Autodesk Inventor part; units mm, degrees
ref_plane "YZ Plane" through (0, 0, 0) normal (1, 0, 0) x (0, 1, 0)
ref_plane "XZ Plane" through (0, 0, 0) normal (0, 1, 0) x (-1, 0, 0)
ref_plane "XY Plane" through (0, 0, 0) normal (0, 0, 1) x (1, 0, 0)
sketch "Sketch1" plane through (0, 0, 0) normal (0, 1, 0) x (-1, 0, 0)
  line L0 (0, 0) -> (0, -71.12)
  line L1 (0, -71.12) -> (71.12, -71.12)
  line L2 (71.12, -71.12) -> (71.12, 0)
  line L3 (71.12, 0) -> (0, 0)
  arc A0 (71.12, -71.12) -> (71.12, 0) centre (-71.8439, -35.56) ccw
  arc A1 (0, 0) -> (0, -71.12) centre (142.9639, -35.56) ccw
  arc A2 (0, -71.12) -> (71.12, -71.12) centre (35.56, 71.8439) ccw
  arc A3 (71.12, 0) -> (0, 0) centre (35.56, -142.9639) ccw
  circle A4 centre (35.56, -35.56) radius 24.13
  dimension "d9" = 71.12
  dimension "d10" = 71.12
  dimension "d14" = 147.32
  dimension "d17" = 48.26
  dimension "d18" = 35.56
  dimension "d19" = 35.56
extrude "Extrusion1" add sketch "Sketch1" along normal blind 3.81
fillet "Fillet1" radius 3.175 4 edges at (0, 1.905, 0) (0, 1.905, -71.12) (-71.12, 1.905, 0) (-71.12, 1.905, -71.12)
sketch "Sketch2" plane through (0, 3.81, 0) normal (0, 1, 0) x (1, 0, 0)
  point P0 (0, 0)
sketch "Sketch3" plane through (0, 0, 0) normal (0, -1, 0) x (1, 0, 0)
  circle A0 centre (-35.56, -35.56) radius 24.13
  circle A1 centre (-35.56, -35.56) radius 31.75
  circle A2 centre (-35.56, -35.56) radius 24.13
  point P0 (0, 0)
  dimension "d23" = 63.5
extrude "Extrusion2" cut sketch "Sketch3" against normal blind 2.1079
sketch "Sketch4" plane through (0, 0, 0) normal (0, -1, 0) x (1, 0, 0)
  circle A0 centre (-35.56, -35.56) radius 24.13
  circle A1 centre (-35.56, -35.56) radius 31.75
  circle A2 centre (-60.96, -10.16) radius 1.905
  arc A3 (-1.9053, 0.4605) -> (-69.2147, 0.4605) centre (-35.56, -142.9639) ccw construction
  line L0 (-35.56, 4.3561) -> (-35.56, -75.4761) construction
  arc A4 (-69.2147, -71.5805) -> (-1.9053, -71.5805) centre (-35.56, 71.8439) ccw construction
  arc A5 (-71.5805, -1.9053) -> (-71.5805, -69.2147) centre (71.8439, -35.56) ccw construction
  line L1 (-75.4761, -35.56) -> (4.3561, -35.56) construction
  arc A6 (0.4605, -69.2147) -> (0.4605, -1.9053) centre (-142.9639, -35.56) ccw construction
  line L2 (-75.4761, -35.56) -> (-75.4761, 1.4435) construction
  circle A7 centre (-10.16, -10.16) radius 1.905
  line L3 (4.3561, -35.56) -> (4.3561, 1.4435) construction
  circle A8 centre (-60.96, -60.96) radius 1.905
  circle A9 centre (-10.16, -60.96) radius 1.905
  point P0 (0, 0)
  dimension "d26" = 3.81
  dimension "d34" = 25.4
  dimension "d35" = 25.4
  dimension "d36" = 14.5161
  dimension "d37" = 14.5162
  dimension "d38" = 50.8
  dimension "d39" = 50.8
extrude "Extrusion3" cut sketch "Sketch4" against normal blind 25.4 contours A2 | A7 | A8 | A9
sketch "Sketch6" plane through (0, 0, 0) normal (0, -1, 0) x (1, 0, 0)
  point P0 (0, 0)
sketch "Sketch8" plane through (0, 3.81, 0) normal (0, 1, 0) x (1, 0, 0)
  circle A0 centre (-35.56, 35.56) radius 24.13
  circle A1 centre (-35.56, 35.56) radius 24.13 construction
  line L0 (-35.56, 59.69) -> (-35.56, 62.23) construction
  line L1 (-35.56, 11.43) -> (-35.56, 8.89) construction
  line L2 (-11.43, 35.56) -> (-8.89, 35.56) construction
  arc A2 (-35.56, 8.89) -> (-35.56, 62.23) centre (-35.56, 35.56) ccw
  line L3 (-35.56, 62.23) -> (-35.56, 8.89)
  point P0 (0, 0)
  dimension "d44" = 2.54
  dimension "d45" = 2.54
  dimension "d46" = 2.54
extrude "Extrusion5" add sketch "Sketch8" along normal blind 2.54 contours A0 L3 | A0 L3 A2 picked at (-28.7553, 42.0502)
fillet "Fillet2" radius 2.54 1 edges at (-8.89, 3.81, -35.56)
properties part number "_3DPrint"
Work out the finished part from the listing and answer in its coordinate system (mm). A direction names the side the tool comes from. Coordinates: 2 decimals unless noted, no trailing zeros. Write each loop counter-clockwise with the first axis right and the second up, starting at its lowest first coordinate (ties: lowest second). Pieces come first, ordered by that corner, then holes.
Q1. A cutting plane is placed at B-B, the plane x = -49. Give the vertices of the cut face in (y, z), then the cut area to 3 significant figures.
Q2. Find the intervals of material crossed by line 1 (X direction, y = 1.5, z = -62); line 2 (Z direction, x = -60.96, y = 2.15) (3 decimals); line 3 (Z direction, x = -10.16, y = 1.1) (3 decimals), in increasing order.
Q3. A cutting plane is placed at C-C, the plane x = -60.96. Give the vertices of the cut face in (y, z) (3 decimals), then the cut area to 3 significant figures.
Q4. Each of these flat-tipped pins is pushed along its axis until it touches: pin 1 Ø12 at (x, z) = (-21, -5) entering from +Y; pin 2 Ø1.3 at (y, z) = (4.5, -32) entering from -X; pin 3 Ø7 at (x, z) = (-20, -32.5) entering from -Y. Where does it stop, or does it pass through?
Q5. Which of the six approach directions +Z, -Z, +X, -X, +Y, -Y give full straight-line access (tool end or side, diameter ignored) to faces 4 (the face through (-35.56, 5, -36)), 5 (the face through (-16.41, 2.95, -20.88)), 6 (the face through (-35.085, 1.878, 4.355))?
Q6. A cutting plane is placed at D-D, the plane y = 5. Give the vertices of the cut face in (x, z).
Q7. Determine the mould class of faces 1 (the face through (-10.41, 1.88, -59.07)), 2 (the face through (4.355, 1.878, -36.035)), 3 (the face through (-53, 3.81, -53)) for opening direction X: released by +X, released by -X, zero draft, split by the parting line, or undercut.
Findings below:
1. outline: (0, -74.86) - (3.81, -74.86) - (3.81, -55.6) - (2.11, -55.6) - (2.11, -64.33) - (0, -64.33) - close; (0, -6.79) - (2.11, -6.79) - (2.11, -15.52) - (3.81, -15.52) - (3.81, 3.74) - (0, 3.74) - close
1. area: 110 mm2
2. line 1: x = -73.08 to -62.56, -59.36 to -53.14, -17.98 to -11.76, -8.56 to 1.96
2. line 2: z = -73.27 to -62.865, -59.055 to -12.065, -8.255 to 2.15
2. line 3: z = -73.27 to -62.865, -59.055 to -54.61, -16.51 to -12.065, -8.255 to 2.15
3. outline: (0, -73.27) - (3.81, -73.27) - (3.81, -62.865) - (0, -62.865) - close; (0, -59.055) - (3.81, -59.055) - (3.81, -12.065) - (0, -12.065) - (0, -16.51) - (2.108, -16.51) - (2.108, -54.61) - (0, -54.61) - close; (0, -8.255) - (3.81, -8.255) - (3.81, 2.15) - (0, 2.15) - close
3. area: 178 mm2
4. pin 1: stops at y = 4.2
4. pin 2: stops at x = -35.56
4. pin 3: stops at y = 3.81
5. face 4: +Z, -Z, -X, +Y
5. face 5: -Y
5. face 6: +Z, +Y, -Y
6. outline: (-35.56, -62.62) arc R27.06 ccw to (-35.56, -8.5) - close
7. face 1: undercut
7. face 2: released by +X
7. face 3: zero draft
